Input: part model. Units: mm. Frame: model coordinates. Face numbers are marked on the shaded views. A direction names the side the tool comes from. Coordinates: 2 decimals unless noted, no trailing zeros. Loops run counter-clockwise (first coordinate to the right, second up) from the corner with the lowest first, then second, coordinate; pieces in that order, holes last. Notation, with made-up numbers: (49, 78.5) - (108, 78.5) arc R9 cw to (108, 83.5) - close; hole circle Ø8 at (16.5, -19). An arc over 180 degrees is marked (long way). Use a Markdown table: item, result. Add a question column.
1. Section query A-A on y = -0.65. Return the cut outline in (x, z), then the cut area to 3 significant figures.
2. Draft query along Z for the marked faces 4, 5 and 6. Return one class per face: released by +Z, released by -Z, zero draft, split by the parting line, or undercut.
3. Section query D-D on x = -8.5. Return the cut outline in (y, z).
4. Access query for the marked faces 1, 2 and 3. Directions: +Z, -Z, +X, -X, +Y, -Y. A direction counts if a zero-diameter tool reaches every point of the face in a straight line with its end or side. Return the directions, or none.
5. Section query C-C on z = 3. Return the cut outline in (x, y).
6. Ray query, L1, parallel to Z at x = 0, y = 1.55; L2, parallel to Z at x = 0.5, y = 0.8; L3, parallel to Y at x = -11, z = -3.5. Return the intervals inside material, ascending. Write a range as [from, to].
7. Contact query for flat-ended pins moving along their axis: P1, Ø1.5, axis at y = 0, z = -4, coming from the -X side; P2, Ø1, axis at x = 17, y = -0.5, coming from the -Z side; P3, Ø5, axis at x = -10.5, z = -20, coming from the -Y side; P4, Ø1, axis at y = -0.5, z = -14.5, coming from the -X side. Output: stop coordinate, or through.
8. Section query B-B on x = 0. Return the cut outline in (y, z), then the cut area to 3 significant figures.
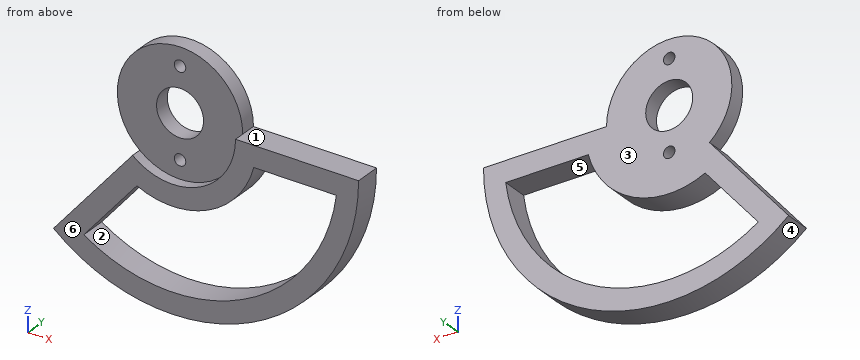
```python
from build123d import *

# Parameters (mm, degrees)
SKETCH1_R           = 12
SKETCH1_R_2         = 4.5
SKETCH1_R_3         = 1.1
BOSS_EXTRUDE1_DEPTH = 3
BOSS_EXTRUDE2_DEPTH = 5
CUT_EXTRUDE1_DEPTH  = 6


with BuildPart() as part:
    # Sketch1 → Boss-Extrude1 (new body)
    with BuildSketch(Plane(origin=(0, 0, 0), x_dir=(1, 0, 0), z_dir=(0, 1, 0))):
        Circle(SKETCH1_R)
        Circle(SKETCH1_R_2, mode=Mode.SUBTRACT)
        with Locations((0, 8.5)):
            Circle(SKETCH1_R_3, mode=Mode.SUBTRACT)
        with Locations((0, -8.5)):
            Circle(SKETCH1_R_3, mode=Mode.SUBTRACT)
    extrude(amount=BOSS_EXTRUDE1_DEPTH)

    # Sketch2 → Boss-Extrude2 (add)
    with BuildSketch(Plane(origin=(0, 3, 0), x_dir=(1, 0, 0), z_dir=(0, 1, 0))):
        with BuildLine():
            Line((12, 0), (35.56, 0))
            ThreePointArc((35.56, 0), (15.028305387, 32.228304907), (-22.8575274, 27.240540397))
            Line((-22.8575274, 27.240540397), (-7.713451316, 9.192533317))
            ThreePointArc((-7.713451316, 9.192533317), (5.071419141, 10.875693444), (12, 0))
        make_face()
    extrude(amount=-BOSS_EXTRUDE2_DEPTH)

    # Sketch3 → Cut-Extrude1 (cut, through all)
    with BuildSketch(Plane.XZ.offset(2)):
        with BuildLine():
            Line((31.305488337, -4), (15.491933385, -4))
            ThreePointArc((15.491933385, -4), (6.761892188, -14.500924593), (-6.893845057, -14.438659921))
            Line((-6.893845057, -14.438659921), (-17.058602246, -26.552545818))
            ThreePointArc((-17.058602246, -26.552545818), (13.337832341, -28.603073759), (31.305488337, -4))
        make_face()
    extrude(amount=-CUT_EXTRUDE1_DEPTH, mode=Mode.SUBTRACT)


solid = part.part
```
Resolved:
| question | item | result |
|---|---|---|
| 1 | outline | (-22.86, -27.24) arc R35.56 ccw to (35.56, 0) - (12, 0) arc R12 cw to (-7.71, -9.19) - close; hole (-17.06, -26.55) arc R31.56 ccw to (31.31, -4) - (15.49, -4) arc R16 cw to (-6.89, -14.44) - close |
| 1 | area | 557 mm² |
| 2 | face 4 | released by -Z |
| 2 | face 5 | undercut |
| 2 | face 6 | zero draft |
| 3 | outline | (-2, -34.53) - (3, -34.53) - (3, -30.39) - (-2, -30.39) - close; (-2, -16.35) - (3, -16.35) - (3, -10.13) - (-2, -10.13) - close; (0, -8.47) - (3, -8.47) - (3, 8.47) - (0, 8.47) - close |
| 4 | face 1 | +Z, +X, +Y, -Y |
| 4 | face 2 | +Y, -Y |
| 4 | face 3 | +Z, -Z, +X, -X, +Y |
| 5 | outline | (-11.62, 0) - (-3.35, 0) - (-3.35, 3) - (-11.62, 3) - close; (3.35, 0) - (11.62, 0) - (11.62, 3) - (3.35, 3) - close |
| 6 | L1 | [-35.56, -31.56], [-16, -9.6], [-7.4, -4.5], [4.5, 7.4], [9.6, 12] |
| 6 | L2 | [-35.56, -31.56], [-15.99, -9.48], [-7.52, -4.47], [4.47, 7.52], [9.48, 11.99] |
| 6 | L3 | [0, 3] |
| 7 | P1 | x = -11.55 |
| 7 | P2 | z = -31.5 |
| 7 | P3 | y = -2 |
| 7 | P4 | x = -12.59 |
| 8 | outline | (-2, -35.56) - (3, -35.56) - (3, -31.56) - (-2, -31.56) - close; (-2, -16) - (3, -16) - (3, -9.6) - (0, -9.6) - (0, -12) - (-2, -12) - close; (0, -7.4) - (3, -7.4) - (3, -4.5) - (0, -4.5) - close; (0, 4.5) - (3, 4.5) - (3, 7.4) - (0, 7.4) - close; (0, 9.6) - (3, 9.6) - (3, 12) - (0, 12) - close |
| 8 | area | 71.8 mm² |
